Source: CAD feature listing. Evaluate the final solid. Frame: model axes, mm. A direction names the side the tool comes from. Coordinates: 2 decimals unless noted, no trailing zeros. Order: outer loops, then holes, each group sorted by start corner. A loop starts at its lowest first (then second) coordinate and runs counter-clockwise, first axis right, second up.
```python
from build123d import *

# Parameters (mm, degrees)
SKETCH1_W           = 280
SKETCH1_H           = 210
BOSS_EXTRUDE1_DEPTH = 15
SKETCH2_R           = 5
BOSS_EXTRUDE2_DEPTH = 50
SKETCH3_W           = 10
SKETCH3_H           = 30
BOSS_EXTRUDE3_DEPTH = 50
SKETCH5_W           = 360.4909063
SKETCH5_H           = 249.182613404
SKETCH5_W_2         = 248.173776912
SKETCH5_H_2         = 125.095724948
CUT_EXTRUDE5_DEPTH  = 15
CUT_EXTRUDE6_START  = -65
SKETCH7_R           = 5
CUT_EXTRUDE6_DEPTH  = 65
SKETCH8_R           = 10
CUT_EXTRUDE7_DEPTH  = 12
SKETCH9_W           = 29.13
SKETCH9_H           = 16.72
CUT_EXTRUDE8_DEPTH  = 15
SKETCH10_W          = 26.78462743
SKETCH10_H          = 41.395526334
CUT_EXTRUDE9_DEPTH  = 27
SKETCH11_W          = 10
SKETCH11_H          = 49
BOSS_EXTRUDE4_DEPTH = 10
SKETCH12_W          = 10
SKETCH12_H          = 49
BOSS_EXTRUDE5_DEPTH = 10
SKETCH4_R           = 13.05
CUT_EXTRUDE10_DEPTH = 74.738133634


with BuildPart() as part:
    # Sketch1 → Boss-Extrude1 (new body)
    with BuildSketch(Plane(origin=(0, 0, 0), x_dir=(1, 0, 0), z_dir=(0, 1, 0))):
        Rectangle(SKETCH1_W, SKETCH1_H)
    extrude(amount=BOSS_EXTRUDE1_DEPTH)

    # Sketch2 → Boss-Extrude2 (add)
    with BuildSketch(Plane(origin=(0, 15, 0), x_dir=(1, 0, 0), z_dir=(0, 1, 0))):
        with Locations(Location((-100, 0, 0), (0, 0, 270))):
            Circle(SKETCH2_R)
        with Locations(Location((-100, 45, 0), (0, 0, 270))):
            Circle(SKETCH2_R)
        with Locations(Location((-100, -45, 0), (0, 0, 270))):
            Circle(SKETCH2_R)
    extrude(amount=BOSS_EXTRUDE2_DEPTH)

    # Sketch3 → Boss-Extrude3 (add)
    with BuildSketch(Plane(origin=(0, 15, 0), x_dir=(1, 0, 0), z_dir=(0, 1, 0))):
        Rectangle(SKETCH3_W, SKETCH3_H)
    extrude(amount=BOSS_EXTRUDE3_DEPTH)

    # Sketch5 → Cut-Extrude5 (cut)
    with BuildSketch(Plane(origin=(0, 0, 0), x_dir=(1, 0, 0), z_dir=(0, 1, 0))):
        with Locations((1.345115322, -3.19464889)):
            Rectangle(SKETCH5_W, SKETCH5_H)
        Rectangle(SKETCH5_W_2, SKETCH5_H_2, mode=Mode.SUBTRACT)
    extrude(amount=CUT_EXTRUDE5_DEPTH, mode=Mode.SUBTRACT)

    # Sketch7 → Cut-Extrude6 (cut)
    with BuildSketch(Plane(origin=(0, 65, 0), x_dir=(1, 0, 0), z_dir=(0, 1, 0)).offset(CUT_EXTRUDE6_START)):
        with Locations(Location((-100, 45, 0), (0, 0, 270))):
            Circle(SKETCH7_R)
        with Locations(Location((-100, 0, 0), (0, 0, 270))):
            Circle(SKETCH7_R)
        with Locations(Location((-100, -45, 0), (0, 0, 270))):
            Circle(SKETCH7_R)
    extrude(amount=CUT_EXTRUDE6_DEPTH, mode=Mode.SUBTRACT)

    # Sketch8 → Cut-Extrude7 (cut)
    with BuildSketch(Plane.XZ):
        with Locations(Location((-100, 45, 0), (0, 0, 270))):
            Circle(SKETCH8_R)
        with Locations(Location((-100, 0, 0), (0, 0, 270))):
            Circle(SKETCH8_R)
        with Locations(Location((-100, -45, 0), (0, 0, 270))):
            Circle(SKETCH8_R)
    extrude(amount=-CUT_EXTRUDE7_DEPTH, mode=Mode.SUBTRACT)

    # Sketch9 → Cut-Extrude8 (cut)
    with BuildSketch(Plane(origin=(0, 15, 0), x_dir=(1, 0, 0), z_dir=(0, 1, 0))):
        with Locations((-48.397782089, 51.271912045)):
            Rectangle(SKETCH9_W, SKETCH9_H)
    extrude(amount=-CUT_EXTRUDE8_DEPTH, mode=Mode.SUBTRACT)

    # Sketch10 → Cut-Extrude9 (cut)
    with BuildSketch(Plane(origin=(0, 15, 0), x_dir=(1, 0, 0), z_dir=(0, 1, 0))):
        Polygon((10.617962241, 62.547862474), (-124.086888456, 62.547862474), (-124.086888456, -62.547862474), (10.617962241, -62.547862474), (124.086888456, -62.547862474), (124.086888456, 62.547862474), align=None)
        with Locations((-5.842214377, 0)):
            Rectangle(SKETCH10_W, SKETCH10_H, mode=Mode.SUBTRACT)
    extrude(amount=-CUT_EXTRUDE9_DEPTH, mode=Mode.SUBTRACT)

    # Sketch11 → Boss-Extrude4 (add)
    with BuildSketch(Plane(origin=(0, 0, -15), x_dir=(-1, 0, 0), z_dir=(0, 0, -1))):
        with Locations((0, 40.5)):
            Rectangle(SKETCH11_W, SKETCH11_H)
    extrude(amount=BOSS_EXTRUDE4_DEPTH)

    # Sketch12 → Boss-Extrude5 (add)
    with BuildSketch(Plane.XY.offset(15)):
        with Locations((0, 40.5)):
            Rectangle(SKETCH12_W, SKETCH12_H)
    extrude(amount=BOSS_EXTRUDE5_DEPTH)

    # Sketch4 → Cut-Extrude10 (cut, through all)
    with BuildSketch(Plane(origin=(5, 0, 0), x_dir=(0, 0, -1), z_dir=(1, 0, 0))):
        with Locations((0, 41.236240869)):
            Circle(SKETCH4_R)
    extrude(amount=-CUT_EXTRUDE10_DEPTH, mode=Mode.SUBTRACT)


solid = part.part
```
Q1. Material intervals for line 1 along Y through (x, z) = (1.25, 0); line 2 along Y through (x, z) = (-6.25, 5.5); line 3 along Z through (x, y) = (-11.5, 8.5), sorted ascending.
Solutions:
line 1: y = 0 to 28.19, 54.29 to 65
line 2: y = 0 to 15
line 3: z = -20.7 to 20.7
Q2. Section query B-B on y = 46.5. Output: boundary loops of the cut face in (x, z).
Solutions:
outline: (-5, -25) - (5, -25) - (5, -11.94) - (-5, -11.94) - close; (-5, 11.94) - (5, 11.94) - (5, 25) - (-5, 25) - close
Q3. Set-up query: faces 1 (the flat face through (0, 16, -20)), 2 (the flat face through (-6, 8, -20.698)), 3 (the flat face through (-6, 8, 20.698)), 4 (the flat face through (5, 29, -6)), 5 (the flat face through (0, 16, 20)). Return all of +Z, -Z, +X, -X, +Y, -Y with unobstructed straight access to the full face (end or side cutting, diameter ignored); none if empty.
Solutions:
face 1: -Z, +X, -X
face 2: -Z, +X, -X, -Y
face 3: +Z, +X, -X, -Y
face 4: +Z, -Z, +X, +Y
face 5: +Z, +X, -X
Q4. Pin query (flat end, axial travel): P1, Ø4, axis at y = 21, z = -9, coming from the -X side; P2, Ø0.8, axis at x = 2, y = 15.5, coming from the -Z side; P3, Ø1.5, axis at y = 27, z = 12.5, coming from the +X side. Return the tip coordinate at first contact, or that it passes through.
Solutions:
P1: stops at x = -5
P2: stops at z = -15
P3: stops at x = 5
Q5. Pull-direction query (Z, two-part tool) for faces 6 (the flat face through (0, 41, 25)), 7 (the cylindrical face through (0.07, 54.175, 1.699)), 8 (the flat face through (-9, 15, 0)), 9 (the flat face through (0, 41, -25)); classes: pulls with the +Z half, pulls with the -Z half, needs draft (parallel to the pull), parting line crosses it, or undercut.
Solutions:
face 6: pulls with the +Z half
face 7: undercut
face 8: needs draft
face 9: pulls with the -Z half
Q6. Section query A-A on z = 0. Output: boundary loops of the cut face in (x, y), plus the area to 3 significant figures.
Solutions:
outline: (-19.23, 0) - (7.55, 0) - (7.55, 15) - (5, 15) - (5, 28.19) - (-5, 28.19) - (-5, 15) - (-19.23, 15) - close; (-5, 54.29) - (5, 54.29) - (5, 65) - (-5, 65) - close
area: 641 mm2
Q7. Section query D-D on y = 12.5. Output: boundary loops of the cut face in (x, z).
Solutions:
outline: (-19.23, -20.7) - (7.55, -20.7) - (7.55, 20.7) - (-19.23, 20.7) - close
Q8. Section query C-C on z = -18.5. Output: boundary loops of the cut face in (x, y), plus the area to 3 significant figures.
Solutions:
outline: (-19.23, 0) - (7.55, 0) - (7.55, 15) - (-19.23, 15) - close; (-5, 16) - (5, 16) - (5, 65) - (-5, 65) - close
area: 892 mm2
